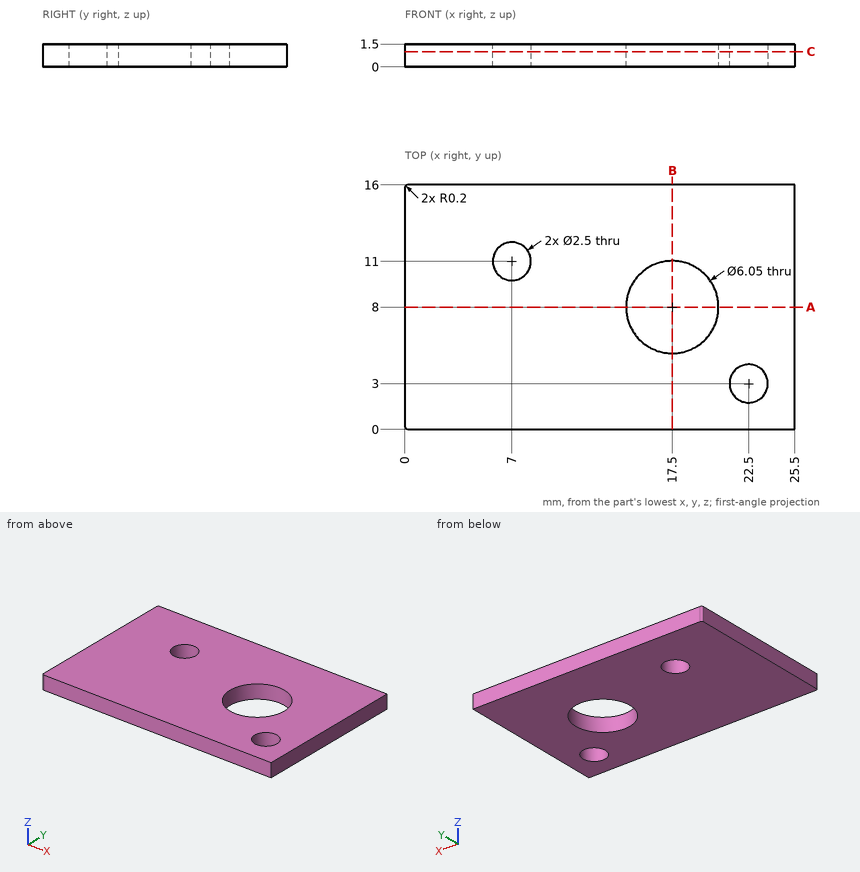
Geometry: see drawing. Coordinates: mm, zero at the bounding-box minimum. Give positions to 0.01 mm unless a question says otherwise; leave off trailing zeros. Order: outer loops, then holes, each group sorted by start corner. A loop starts at its lowest first (then second) coordinate and runs counter-clockwise, first axis right, second up. Notation, with made-up numbers: (13.25, -36.75) - (38.25, -36.75) arc R13 cw to (38.25, -21.75) - close; hole circle Ø4 at (25, -15). An arc over 180 degrees is marked (long way). Write each question's results on one line, items separated by ' | '.
Item 1: Section B-B (x = 17.5). Return loops of the section in (y, z) (3 decimals), and give its area (3 significant figures).
A:
outline: (0, 0) - (4.975, 0) - (4.975, 1.5) - (0, 1.5) - close; (11.025, 0) - (16, 0) - (16, 1.5) - (11.025, 1.5) - close | area: 14.9 mm^2
Item 2: Material intervals for line 1 along Y through (x, z) = (22.5, 0.95); line 2 along X through (y, z) = (10.5, 0.1); line 3 along Y through (x, z) = (17.5, 0.55) (3 decimals), sorted ascending.
A:
line 1: y = 0 to 1.75, 4.25 to 16 | line 2: x = 0 to 5.85, 8.15 to 15.8, 19.2 to 25.5 | line 3: y = 0 to 4.975, 11.025 to 16
Item 3: Section C-C (z = 1). Return loops of the section in (x, y) (3 decimals).
A:
outline: (0, 0.2) arc R0.2 ccw to (0.2, 0) - (25.5, 0) - (25.5, 16) - (0.2, 16) arc R0.2 ccw to (0, 15.8) - close; hole circle Ø2.5 at (7, 11); hole circle Ø6.05 at (17.5, 8); hole circle Ø2.5 at (22.5, 3)
Item 4: Section A-A (y = 8). Return loops of the section in (x, z) (3 decimals), and give its area (3 significant figures).
A:
outline: (0, 0) - (14.475, 0) - (14.475, 1.5) - (0, 1.5) - close; (20.525, 0) - (25.5, 0) - (25.5, 1.5) - (20.525, 1.5) - close | area: 29.2 mm^2
Item 5: Contact query for flat-ended pins moving along their axis: pin 1 Ø9.5 at (x, y) = (17.5, 8) entering from +Z; pin 2 Ø2 at (x, y) = (7, 11) entering from -Z. Output: stop coordinate, or through.
A:
pin 1: stops at z = 1.5 | pin 2: passes through
